Read the model definition and answer for the solid it produces. Units are mm, in the model's axes. A direction names the side the tool comes from. Coordinates: 2 decimals unless noted, no trailing zeros. Order: outer loops, then holes, each group sorted by start corner. A loop starts at its lowest first (then second) coordinate and runs counter-clockwise, first axis right, second up. Notation, with made-up numbers: (-1, 67) - (4, 67) arc R23 ccw to (4, 76) - close; hole circle Ø3 at (-34.75, -33.75). An arc over 180 degrees is marked (long way). Answer as a JSON object with one key per item and string values. Group by question number.
from build123d import *

# Parameters (mm, degrees)
F0_R     = 1.5
F1_DEPTH = 3
F3_DEPTH = 4
F4_R     = 1.5
F5_DEPTH = 20


with BuildPart() as f1:
    # F0 (on Front) → F1 (new body)
    with BuildSketch(Plane.XZ):
        with BuildLine():
            Line((5.9394528039, 2.640625), (2.9697264019, 9.3203125))
            ThreePointArc((2.9697264019, 9.3203125), (0, 11.25), (-2.9697264019, 9.3203125))
            Line((-2.9697264019, 9.3203125), (-5.9394528039, 2.640625))
            ThreePointArc((-5.9394528039, 2.640625), (0, -6.5), (5.9394528039, 2.640625))
        make_face()
        with Locations((0, 8)):
            Circle(F0_R, mode=Mode.SUBTRACT)
    extrude(amount=-F1_DEPTH)

    # F2 (on face) → F3 (join)
    with BuildSketch(Plane.XZ):
        with BuildLine():
            ThreePointArc((-2.0615528128, 4), (-2.3423292192, -3.8423292192), (4.5, 0))
            ThreePointArc((4.5, 0), (3.8423292192, 2.3423292192), (2.0615528128, 4))
            Line((2.0615528128, 4), (-2.0615528128, 4))
        make_face()
    extrude(amount=F3_DEPTH)

    # F4 (on face) → F5 (cut)
    with BuildSketch(Plane.XZ.offset(4)):
        Circle(F4_R)
    extrude(amount=-F5_DEPTH, mode=Mode.SUBTRACT)


solid = f1.part
1. Straight lines are drawn through the part: L1, parallel to Z at x = 0, y = 0.9; L2, parallel to Z at x = 0, y = -0.25; L3, parallel to Y at x = 4.25, z = -3.5. For each, find the intervals that lie inside material, in ascending order.
2. A cutting plane is placed at D-D on y = 2.5. Write down the section's boundary in (x, z).
3. A cutting plane is placed at A-A on x = 0. Write down the section's boundary in (y, z), and give its area (4 significant figures).
4. A cutting plane is placed at B-B on z = 8. Write down the section's boundary in (x, y), and give its area (3 significant figures).
5. For a pull along Z with two mould halves and no side action, classify faces 1 (the flat face through (0, -4, 2)), 2 (the cylindrical face through (-1.5, -0.55, 0.07)), 3 (the flat face through (0, -2, 4)) as pulls with the +Z half, pulls with the -Z half, needs draft (parallel to the pull), parting line crosses it, or undercut.
6. Given pin 1 (4 mm diameter, centred on y = -0.5, z = 3, fed in from -X); pin 2 (2 mm diameter, centred on y = 1.5, z = 1.5, fed in from -X); pin 3 (5 mm diameter, centred on x = 0, z = 8, fed in from -Y); pin 4 (4 mm diameter, centred on x = 0, z = 0, fed in from -Y), each flat-ended and moving along its own axis, determine where each tip first touches the part or whether it passes through.
7. A cutting plane is placed at C-C on y = -2. Write down the section's boundary in (x, z).
8. For faces 4 (the flat face through (-0.1, 0, 4.5)), 5 (the flat face through (4.475, 1.479, 5.934)), determine the directions among +Z, -Z, +X, -X, +Y, -Y from which every point of the face is accessible in a straight line to the end or side of a thin tool.
Derived:
{
 "1": {"L1": "z = -6.5 to -1.5, 1.5 to 6.5, 9.5 to 11.25", "L2": "z = -4.5 to -1.5, 1.5 to 4", "L3": "y = 0 to 3"},
 "2": {"outline": "(-5.94, 2.64) arc R6.5 ccw (long way) to (5.94, 2.64) - (2.97, 9.32) arc R3.25 ccw to (-2.97, 9.32) - close; hole circle Ø3 at (0, 0); hole circle Ø3 at (0, 8)"},
 "3": {"outline": "(-4, -4.5) - (0, -4.5) - (0, -6.5) - (3, -6.5) - (3, -1.5) - (-4, -1.5) - close; (-4, 1.5) - (3, 1.5) - (3, 6.5) - (0, 6.5) - (0, 4) - (-4, 4) - close; (0, 9.5) - (3, 9.5) - (3, 11.25) - (0, 11.25) - close", "area": "57.25 mm2"},
 "4": {"outline": "(-3.56, 0) - (-1.5, 0) - (-1.5, 3) - (-3.56, 3) - close; (1.5, 0) - (3.56, 0) - (3.56, 3) - (1.5, 3) - close", "area": "12.3 mm2"},
 "5": {"face 1": "needs draft", "face 2": "undercut", "face 3": "pulls with the +Z half"},
 "6": {"pin 1": "stops at x = -6.41", "pin 2": "stops at x = -6.48", "pin 3": "stops at y = 0", "pin 4": "stops at y = -4"},
 "7": {"outline": "(-2.06, 4) arc R4.5 ccw (long way) to (2.06, 4) - close; hole circle Ø3 at (0, 0)"},
 "8": {"face 4": "-Y", "face 5": "+Z, +X, +Y, -Y"}
}
